```python
from build123d import *

# Parameters (mm, degrees)
SKETCH1_W           = 30.5
SKETCH1_H           = 62
BOSS_EXTRUDE1_DEPTH = 12
CUT_EXTRUDE1_START  = -46
CUT_EXTRUDE1_DEPTH  = 46


with BuildPart() as part:
    # Sketch1 → Boss-Extrude1 (new body)
    with BuildSketch(Plane(origin=(0, 0, 0), x_dir=(1, 0, 0), z_dir=(0, 1, 0))):
        Rectangle(SKETCH1_W, SKETCH1_H)
    extrude(amount=BOSS_EXTRUDE1_DEPTH)

    # Sketch2 → Cut-Extrude1 (cut)
    with BuildSketch(Plane(origin=(0, 0, -23), x_dir=(-1, 0, 0), z_dir=(0, 0, -1)).offset(CUT_EXTRUDE1_START)):
        Polygon((-15.25, 12), (15.25, 12), (-15.25, 2.089949265), align=None)
    extrude(amount=CUT_EXTRUDE1_DEPTH, mode=Mode.SUBTRACT)


solid = part.part
```
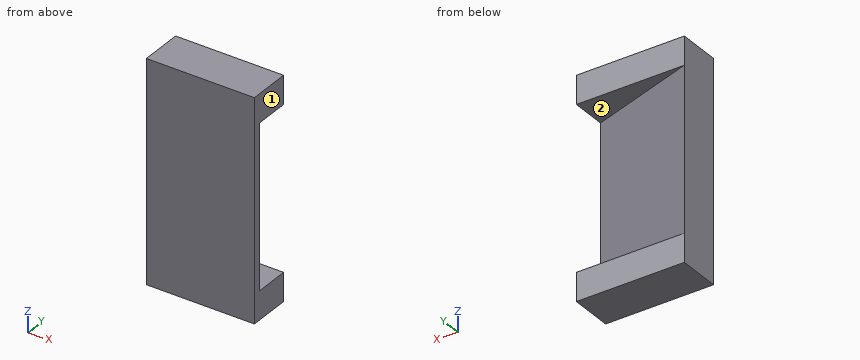
Source: CAD feature listing. Evaluate the final solid. Frame: model axes, mm. Face numbers are marked on the shaded views. A direction names the side the tool comes from. Coordinates: 2 decimals unless noted, no trailing zeros. Loops run counter-clockwise (first coordinate to the right, second up) from the corner with the lowest first, then second, coordinate; pieces in that order, holes last. Notation, with made-up numbers: (6.25, 5) -> (24.25, 5) arc R9 ccw to (24.25, 13) -> close; hole circle Ø5 at (88.5, 54.25). An arc over 180 degrees is marked (long way). One line per item, written item: value. Start each with the question number.
Q1. Section query A-A, the plane x = -5.5. Return the cut outline in (y, z).
Q2. Line query: line 1 along Z through (x, y) = (9.5, 10.25); line 2 along Y through (x, z) = (-12, -17.5); line 3 along Y through (x, z) = (11, 12.5). Output: solid intervals per line, ascending.
Q3. Set-up query: the marked faces 1 and 2. Return all of +Z, -Z, +X, -X, +Y, -Y with unobstructed straight access to the full face (end or side cutting, diameter ignored); none if empty.
Q4. Section query B-B, the plane y = 10.5. Return the cut outline in (x, z).
Q5. Section query C-C, the plane z = -3.5. Return the cut outline in (x, y).
Q6. Contact query for flat-ended pins moving along their axis: P1, Ø10, axis at x = 2, z = 14.5, coming from the +Y side; P2, Ø6, axis at x = -9.5, z = -9.5, coming from the +Y side; P3, Ø1, axis at x = -11.5, z = -9, coming from the +Y side. Output: stop coordinate, or through.
Results:
1. outline: (0, -31) -> (12, -31) -> (12, -23) -> (8.83, -23) -> (8.83, 23) -> (12, 23) -> (12, 31) -> (0, 31) -> close
2. line 1: -31 to -23, 23 to 31
2. line 2: 0 to 10.94
2. line 3: 0 to 3.47
3. face 1: +Z, -Z, +X, +Y, -Y
3. face 2: +X, +Y
4. outline: (-15.25, -31) -> (15.25, -31) -> (15.25, -23) -> (-10.63, -23) -> (-10.63, 23) -> (15.25, 23) -> (15.25, 31) -> (-15.25, 31) -> close
5. outline: (-15.25, 0) -> (15.25, 0) -> (15.25, 2.09) -> (-15.25, 12) -> close
6. P1: y = 8.02
6. P2: y = 11.11
6. P3: y = 10.94
